The model under review builds one solid part; all positions refer to its coordinate system, in mm. Face numbers are marked on the shaded views. A direction names the side the tool comes from. Round coordinates to 2 decimals unless told otherwise and drop trailing zeros. Order: outer loops, then holes, each group sorted by start corner. A loop starts at its lowest first (then second) coordinate and runs counter-clockwise, first axis right, second up. Notation, with made-up numbers: M 23.5,11.5 L 71.5,11.5 A27 ccw 71.5,43.5 Z; hole C 12,-14 d6. An arc over 180 degrees is marked long. Answer as a JSON object with one key per item and string values. Group by question number.
1. Machinability: for the marked faces 1, 2 and 3, which of the approach directions +Z, -Z, +X, -X, +Y, -Y give a long, thin tool a straight path to every point of the face, cutting with its end or side? Answer none if there is none.
2. Clearance check with flat-ended pins moving along their axes: P1, Ø3, axis at x = -7, z = -7.5, coming from the +Y side; P2, Ø4, axis at y = 106.16, z = -5, coming from the -X side; P3, Ø4, axis at x = -8, z = -4.5, coming from the +Y side. State where each tip first meets the part, or that it passes through.
3. To check wall thickness, follow probe 1 along X at (y, z) = (-32, -5.5); probe 2 along X at (y, z) = (62, -6); probe 3 along Y at (x, z) = (-1, -5). State the ranges of each line that lie inside material, in increasing order. Write a range as [from, to].
4. Add section B-B on y = 35. State the section outline as (x, z) points.
5. Add section C-C on x = -3.25. State the section outline as (y, z) points, and give its area (3 significant figures).
6. Add section A-A on z = -5. State the section outline as (x, y) points.
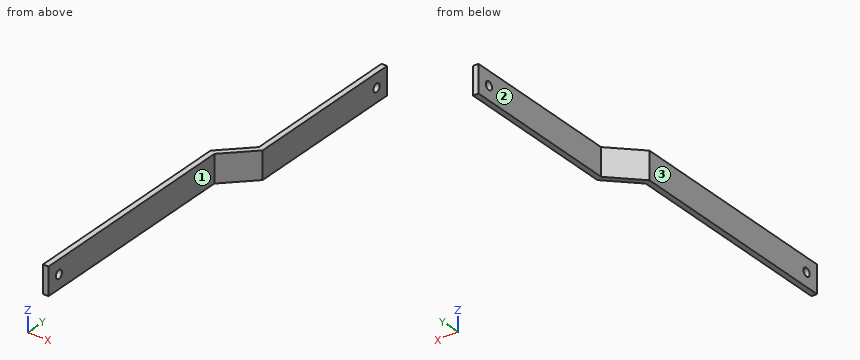
Autodesk Inventor part; units mm, degrees
ref_plane "YZ Plane" through (0, 0, 0) normal (1, 0, 0) x (0, 1, 0)
ref_plane "XZ Plane" through (0, 0, 0) normal (0, 1, 0) x (-1, 0, 0)
ref_plane "XY Plane" through (0, 0, 0) normal (0, 0, 1) x (1, 0, 0)
sketch "Skizze1" plane through (0, 0, 0) normal (0, 0, 1) x (1, 0, 0)
  line L0 (-14.4, 0) -> (2.4, 0)
  line L1 (0, -68.8373) -> (0, 141.1627)
  line L2 (-10, -38.8373) -> (-10, 41.1627)
  line L3 (-10, 41.1627) -> (0, 51.1627)
  line L4 (0, 51.1627) -> (0, 111.1627)
  line L5 (-10, -38.8373) -> (-12, -38.8373)
  line L6 (-12, -38.8373) -> (-12, 41.9912)
  line L7 (-2, 51.9912) -> (-12, 41.9912)
  line L8 (-2, 111.1627) -> (0, 111.1627)
  line L9 (-2, 111.1627) -> (-2, 51.9912)
  point P0 (0, 0)
  dimension "d0" = 80
  dimension "d2" = 60
  dimension "d5" = 2
  dimension "d6" = 2
  dimension "d7" = 2
  dimension "d20" = 10
  dimension "d22" = 150
extrude "Extrusion1" add sketch "Skizze1" against normal blind 10 contours L6 L7 L9 L8 L1 L3 L2 L0 | L0 L2 L5 L6
sketch "Skizze2" plane through (-12, -38.8373, 0) normal (-1, 0, 0) x (0, 0, 1)
  line L0 (0, 80.8284) -> (0, 0)
  line L1 (0, 0) -> (-10, 0)
  circle A0 centre (-5, 5) radius 1.5
  point P0 (0, 38.8373)
  dimension "d10" = 5
  dimension "d11" = 5
  dimension "d12" = 3
extrude "Extrusion2" cut sketch "Skizze2" against normal blind 5
sketch "Skizze3" plane through (-2, 51.9912, 0) normal (-1, 0, 0) x (0, 0, 1)
  line L0 (-10, 0) -> (-10, 59.1716)
  line L1 (0, 59.1716) -> (-10, 59.1716)
  circle A0 centre (-5, 54.1716) radius 1.5
  point P0 (0, -51.9912)
  dimension "d15" = 5
  dimension "d16" = 5
  dimension "d17" = 3
extrude "Extrusion3" cut sketch "Skizze3" against normal blind 5
properties part number "Gestänge"
Recorded:
{
 "1": {"face 1": "+Z, -Z, +X, -Y", "face 2": "+Z, -Z, -X, +Y", "face 3": "+Z, -Z, -X, +Y, -Y"},
 "2": {"P1": "stops at y = 48.49", "P2": "stops at x = -2", "P3": "stops at y = 47.99"},
 "3": {"probe 1": "x = [-12, -10]", "probe 2": "x = [-2, 0]", "probe 3": "y = [50.16, 104.66], [107.66, 111.16]"},
 "4": {"outline": "M -12,-10 L -10,-10 L -10,0 L -12,0 Z"},
 "5": {"outline": "M 47.91,-10 L 50.74,-10 L 50.74,0 L 47.91,0 Z", "area": "28.3 mm²"},
 "6": {"outline": "M -12,-38.84 L -10,-38.84 L -10,-35.34 L -12,-35.34 Z; M -12,-32.34 L -10,-32.34 L -10,41.16 L 0,51.16 L 0,104.66 L -2,104.66 L -2,51.99 L -12,41.99 Z; M -2,107.66 L 0,107.66 L 0,111.16 L -2,111.16 Z"}
}
